Input: part model. Units: mm. Frame: model coordinates. A direction names the side the tool comes from. Give positions to 0.01 mm unless a question says otherwise; leave off trailing zeros. Order: outer loops, then holes, each group sorted by start corner. A loop starts at its lowest first (then second) coordinate and runs counter-clockwise, first axis right, second up.
```python
from build123d import *

# Parameters (mm, degrees)
BOSS_EXTRUDE1_DEPTH = 3
SKETCH8_R           = 1.05
CUT_EXTRUDE1_DEPTH  = 28.739863013
SKETCH9_R           = 7.5
CUT_EXTRUDE2_DEPTH  = 2
SKETCH10_W          = 5
SKETCH10_H          = 4.5
SKETCH10_W_2        = 4.5
SKETCH10_H_2        = 5
BOSS_EXTRUDE2_DEPTH = 5
SKETCH11_R          = 0.6
CUT_EXTRUDE3_DEPTH  = 6
CUT_EXTRUDE4_DEPTH  = 3.5
CIRPATTERN1_COUNT   = 4
SKETCH15_W          = 3.5
SKETCH15_H          = 1.8
CUT_EXTRUDE5_DEPTH  = 4.2
CIRPATTERN2_COUNT   = 4
SKETCH16_W          = 14.5
SKETCH16_H          = 14.5
CUT_EXTRUDE6_DEPTH  = 2
FILLET1_R           = 0.4
SKETCH17_W          = 14
SKETCH17_H          = 14
BOSS_EXTRUDE3_DEPTH = 14
SKETCH18_W          = 54
SKETCH18_H          = 11
BOSS_EXTRUDE4_DEPTH = 6.5


with BuildPart() as part:
    # Sketch1 → Boss-Extrude1 (new body)
    with BuildSketch(Plane(origin=(0, 0, 0), x_dir=(1, 0, 0), z_dir=(0, 1, 0))):
        Polygon((19.5, -15), (19.5, -10), (15, -10), (15, 19.5), (10, 19.5), (10, 15), (-19.5, 15), (-19.5, 10), (-15, 10), (-15, -19.5), (-10, -19.5), (-10, -15), align=None)
    extrude(amount=BOSS_EXTRUDE1_DEPTH)

    # Sketch8 → Cut-Extrude1 (cut, through all)
    with BuildSketch(Plane(origin=(0, 0, 0), x_dir=(-1, 0, 0), z_dir=(0, -1, 0))):
        with Locations(Location((-12.75, 12.75, 0), (0, 0, 90))):
            Circle(SKETCH8_R)
        with Locations(Location((12.75, 12.75, 0), (0, 0, 90))):
            Circle(SKETCH8_R)
        with Locations(Location((12.75, -12.75, 0), (0, 0, 90))):
            Circle(SKETCH8_R)
        with Locations(Location((-12.75, -12.75, 0), (0, 0, 90))):
            Circle(SKETCH8_R)
    extrude(amount=-CUT_EXTRUDE1_DEPTH, mode=Mode.SUBTRACT)

    # Sketch9 → Cut-Extrude2 (cut)
    with BuildSketch(Plane(origin=(0, 0, 0), x_dir=(-1, 0, 0), z_dir=(0, -1, 0))):
        with Locations(Location((0, 0, 0), (0, 0, 90))):
            Circle(SKETCH9_R)
    extrude(amount=-CUT_EXTRUDE2_DEPTH, mode=Mode.SUBTRACT)

    # Sketch10 → Boss-Extrude2 (add)
    with BuildSketch(Plane.XZ):
        with Locations((-12.5, 17.25)):
            Rectangle(SKETCH10_W, SKETCH10_H)
        with Locations((-17.25, -12.5)):
            Rectangle(SKETCH10_W_2, SKETCH10_H_2)
        with Locations((12.5, -17.25)):
            Rectangle(SKETCH10_W, SKETCH10_H)
        with Locations((17.25, 12.5)):
            Rectangle(SKETCH10_W_2, SKETCH10_H_2)
    extrude(amount=BOSS_EXTRUDE2_DEPTH)

    # Sketch11 → Cut-Extrude3 (cut)
    with BuildSketch(Plane.XZ.offset(5)):
        with Locations(Location((-12.5, 17.25, 0), (0, 0, 270))):
            Circle(SKETCH11_R)
    cut_extrude3 = extrude(amount=-CUT_EXTRUDE3_DEPTH, mode=Mode.SUBTRACT)

    # Sketch13 → Cut-Extrude4 (cut)
    with BuildSketch(Plane(origin=(0, 0, 15), x_dir=(-1, 0, 0), z_dir=(0, 0, -1))):
        Polygon((10.85, -3.4), (14.15, -3.4), (15, -3.4), (15, -1.6), (14.15, -1.6), (10.85, -1.6), align=None)
    cut_extrude4 = extrude(amount=-CUT_EXTRUDE4_DEPTH, mode=Mode.SUBTRACT)

    # CirPattern1: Cut-Extrude3, Cut-Extrude4 ×4 about axis
    cirpattern1_axis = Axis((0, 0, 0), (0, 1, 0))
    add([cut_extrude3.rotate(cirpattern1_axis, i * 360 / CIRPATTERN1_COUNT) for i in range(1, CIRPATTERN1_COUNT)], mode=Mode.SUBTRACT)
    add([cut_extrude4.rotate(cirpattern1_axis, i * 360 / CIRPATTERN1_COUNT) for i in range(1, CIRPATTERN1_COUNT)], mode=Mode.SUBTRACT)

    # Sketch15 → Cut-Extrude5 (cut)
    with BuildSketch(Plane.XY.offset(15)):
        with Locations((16.75, -2.5)):
            Rectangle(SKETCH15_W, SKETCH15_H)
    cut_extrude5 = extrude(amount=-CUT_EXTRUDE5_DEPTH, mode=Mode.SUBTRACT)

    # CirPattern2: Cut-Extrude5 ×4 about axis
    cirpattern2_axis = Axis((0, 0, 0), (0, 1, 0))
    for i in range(1, CIRPATTERN2_COUNT):
        add(cut_extrude5.rotate(cirpattern2_axis, i * 360 / CIRPATTERN2_COUNT), mode=Mode.SUBTRACT)

    # Sketch16 → Cut-Extrude6 (cut)
    with BuildSketch(Plane.XZ):
        Rectangle(SKETCH16_W, SKETCH16_H)
    extrude(amount=-CUT_EXTRUDE6_DEPTH, mode=Mode.SUBTRACT)

    # Fillet1
    fillet1_edges = [part.edges().sort_by_distance(p)[0] for p in [
        (7.25, 1, 7.25),
        (7.25, 1, -7.25),
        (-7.25, 1, -7.25),
        (-7.25, 1, 7.25),
    ]]
    fillet(fillet1_edges, radius=FILLET1_R)

    # Sketch17 → Boss-Extrude3 (add)
    with BuildSketch(Plane.XZ.offset(-2)):
        Rectangle(SKETCH17_W, SKETCH17_H)
    extrude(amount=BOSS_EXTRUDE3_DEPTH)

    # Sketch18 → Boss-Extrude4 (add)
    with BuildSketch(Plane(origin=(0, 3, 0), x_dir=(1, 0, 0), z_dir=(0, 1, 0))):
        Rectangle(SKETCH18_W, SKETCH18_H)
    extrude(amount=BOSS_EXTRUDE4_DEPTH)


solid = part.part
```
1) Reachability of faces 5 (the face through (21, 3, 0)), 6 (the face through (13, -2, -18.5)), 7 (the face through (16, -1.6, 13)), 8 (the face through (-13, -1.6, 16)), 9 (the face through (-4, 1, -7.25)) from +Z, -Z, +X, -X, +Y, -Y: full face, straight path, thin tool, end or side. Return the list, or none.
2) Cut plane B-B (x = -5). Return the cut outline in (y, z).
3) Cut plane C-C (y = 8). Return the cut outline in (x, z).
4) First-contact query: P1, Ø4, axis at y = -1, z = 15.5, coming from the -X side; P2, Ø6, axis at y = 5, z = -9, coming from the -X side; P3, Ø4, axis at x = -3.5, y = 1, coming from the -Z side. Flat tips, straight axial feed; report the tip coordinate or a pass-through.
5) Pull-direction query (Z, two-part tool) for faces 1 (the face through (16.97, -4.21, 13.03)), 2 (the face through (0, -12, 0)), 3 (the face through (17.3, 1, 12.5)), 4 (the face through (-17, -2, -10.8)); classes: pulls with the +Z half, pulls with the -Z half, needs draft (parallel to the pull), parting line crosses it, or undercut.
6) Cut plane A-A (x = 17.25). Return the cut outline in (y, z).
7) Line query: probe 1 along X at (y, z) = (2, 12.75); probe 2 along X at (y, z) = (1.5, -12.75); probe 3 along X at (y, z) = (-0.95, 17.25). Output: solid intervals per line, ascending.
Geometry says:
1. face 5: -Z, +X, -Y
1. face 6: +Z, +X
1. face 7: +Z, -X
1. face 8: -Z, -X
1. face 9: -Y
2. outline: (-12, -7) - (2, -7) - (2, -7.25) - (0, -7.25) - (0, -15) - (3, -15) - (3, -5.5) - (9.5, -5.5) - (9.5, 5.5) - (3, 5.5) - (3, 15) - (0, 15) - (0, 7.25) - (2, 7.25) - (2, 7) - (-12, 7) - close
3. outline: (-27, -5.5) - (27, -5.5) - (27, 5.5) - (-27, 5.5) - close
4. P1: stops at x = -15
4. P2: stops at x = -19.5
4. P3: stops at z = -15
5. face 1: undercut
5. face 2: needs draft
5. face 3: undercut
5. face 4: pulls with the -Z half
6. outline: (-5, 10) - (3, 10) - (3, 15) - (-1.6, 15) - (-1.6, 13.1) - (1, 13.1) - (1, 11.9) - (-1.6, 11.9) - (-1.6, 10.8) - (-3.4, 10.8) - (-3.4, 11.9) - (-5, 11.9) - close; (-5, 13.1) - (-3.4, 13.1) - (-3.4, 15) - (-5, 15) - close; (3, -5.5) - (9.5, -5.5) - (9.5, 5.5) - (3, 5.5) - close
7. probe 1: x = -15 to -13.8, -11.7 to 11.7, 13.8 to 19.5
7. probe 2: x = -19.5 to -13.8, -11.7 to 11.7, 13.8 to 15
7. probe 3: x = -15 to -13.1, -11.9 to -10
